```python
from build123d import *

# Parameters (mm, degrees)
BOSS_EXTRUDE1_DEPTH      = 12
BOSS_EXTRUDE1_DEPTH_BACK = 2
CUT_EXTRUDE1_DEPTH       = 5
SKETCH5_R                = 1
CUT_EXTRUDE2_DEPTH       = 7.26
CUT_EXTRUDE2_DEPTH_BACK  = 8.74
SKETCH6_R                = 1.95
CUT_EXTRUDE3_DEPTH       = 1.55
CUT_EXTRUDE4_DEPTH       = 2.5


with BuildPart() as part:
    # Sketch1 → Boss-Extrude1 (new body, two sides)
    with BuildSketch(Plane(origin=(0, 0, 0), x_dir=(1, 0, 0), z_dir=(0, 1, 0))) as boss_extrude1_sk:
        with BuildLine():
            Line((4.642363604, -4.565370009), (-4.68242218, -4.565370009))
            Line((-4.68242218, -4.565370009), (-2.520029288, -11.638238463))
            Line((-2.520029288, -11.638238463), (-2.520029288, -16.559323376))
            ThreePointArc((-2.520029288, -16.559323376), (-1.744780523, -16.658855879), (-0.965732534, -16.722114069))
            Line((-0.965732534, -16.722114069), (-0.020029288, -19.815370009))
            Line((-0.020029288, -19.815370009), (0.924969464, -16.724418368))
            ThreePointArc((0.924969464, -16.724418368), (1.704326405, -16.663043233), (2.479970712, -16.565370009))
            Line((2.479970712, -16.565370009), (2.479970712, -11.638238463))
            Line((2.479970712, -11.638238463), (4.642363604, -4.565370009))
        make_face()
    extrude(amount=BOSS_EXTRUDE1_DEPTH)
    extrude(boss_extrude1_sk.sketch, amount=-BOSS_EXTRUDE1_DEPTH_BACK)

    # Sketch2 → Cut-Extrude1 (cut)
    with BuildSketch(Plane(origin=(0, 0, 4.565370009), x_dir=(-1, 0, 0), z_dir=(0, 0, -1))):
        with BuildLine():
            Line((-2.878246061, 5.95), (2.918304637, 5.95))
            ThreePointArc((2.918304637, 5.95), (0.020029288, 8.05), (-2.878246061, 5.95))
        make_face()
        with BuildLine():
            Line((-2.878246061, 4.05), (2.918304637, 4.05))
            ThreePointArc((2.918304637, 4.05), (0.020029288, 1.95), (-2.878246061, 4.05))
        make_face()
    extrude(amount=-CUT_EXTRUDE1_DEPTH, mode=Mode.SUBTRACT)

    # Sketch5 → Cut-Extrude2 (cut, two sides)
    with BuildSketch(Plane(origin=(0, 5.74, 0), x_dir=(1, 0, 0), z_dir=(0, 1, 0))) as cut_extrude2_sk:
        with Locations((0, -7.065370009)):
            Circle(SKETCH5_R)
    extrude(amount=CUT_EXTRUDE2_DEPTH, mode=Mode.SUBTRACT)
    extrude(cut_extrude2_sk.sketch, amount=-CUT_EXTRUDE2_DEPTH_BACK, mode=Mode.SUBTRACT)

    # Sketch6 → Cut-Extrude3 (cut)
    with BuildSketch(Plane(origin=(0, 12, 0), x_dir=(1, 0, 0), z_dir=(0, 1, 0))):
        with Locations((0, -7.065370009)):
            Circle(SKETCH6_R)
    extrude(amount=-CUT_EXTRUDE3_DEPTH, mode=Mode.SUBTRACT)

    # Sketch7 → Cut-Extrude4 (cut)
    with BuildSketch(Plane(origin=(0, 12, 0), x_dir=(1, 0, 0), z_dir=(0, 1, 0))):
        Polygon((0.924969464, -16.724418368), (-0.020029288, -19.815370009), (-0.965732534, -16.722114069), align=None)
    cut_extrude4 = extrude(amount=-CUT_EXTRUDE4_DEPTH, mode=Mode.SUBTRACT)

    # Mirror1: Cut-Extrude4 across plane
    add(cut_extrude4.mirror(Plane.ZX.offset(5)), mode=Mode.SUBTRACT)


solid = part.part
```
Could you check a few things on this model? Use its own coordinates, in mm. A direction names the side the tool comes from. Round coordinates to 2 decimals unless told otherwise and drop trailing zeros. Loops run counter-clockwise (first coordinate to the right, second up) from the corner with the lowest first, then second, coordinate; pieces in that order, holes last. Notation, with made-up numbers: (59.5, -12.5) - (93.5, -12.5) arc R29 cw to (93.5, 9.5) - close; hole circle Ø4 at (-10.5, 88.5). An arc over 180 degrees is marked (long way). Answer as CSV lines item,"result".
1. I want a section at C-C on x = -1.25. List the corners of the cut face in (y, z) for me.
Filled in:
outline,"(-2, 4.57) - (2.21, 4.57) - (2.21, 9.57) - (4.05, 9.57) - (4.05, 4.57) - (5.95, 4.57) - (5.95, 9.57) - (7.79, 9.57) - (7.79, 4.57) - (12, 4.57) - (12, 5.57) - (10.45, 5.57) - (10.45, 8.56) - (12, 8.56) - (12, 16.7) - (-2, 16.7) - close"
2. I want a section at A-A on z = 9.25. List the corners of the cut face in (x, y) for me, then the cut area to 3 significant figures.
Filled in:
outline,"(-3.25, -2) - (3.21, -2) - (3.21, 12) - (-3.25, 12) - close; hole (-2.92, 4.05) arc R3.05 ccw to (2.88, 4.05) - close; hole (-2.92, 5.95) - (2.88, 5.95) arc R3.05 ccw to start"
area,"72.6 mm^2"
3. On a 3-axis mill with a long thin cutter (end or side, diameter ignored), from which of +Z, -Z, +X, -X, +Y, -Y can I reach the whole of each face in a straight line? I mean faces 1 (the face through (-0.42, 11.24, 8.97)), 2 (the face through (0, 3, 9.565)), 3 (the face through (2.48, 5, 14)). Say none if no direction works.
Filled in:
face 1,"+Y"
face 2,"-Z"
face 3,"+Z, +X, +Y, -Y"
4. I want a section at D-D on y = 6.5. List the corners of the cut face in (x, z) for me.
Filled in:
outline,"(-4.68, 4.57) - (-2.68, 4.57) - (-2.68, 9.57) - (2.64, 9.57) - (2.64, 4.57) - (4.64, 4.57) - (2.48, 11.64) - (2.48, 16.57) arc R16.75 ccw to (0.92, 16.72) - (-0.02, 19.82) - (-0.97, 16.72) arc R16.75 ccw to (-2.52, 16.56) - (-2.52, 11.64) - close"
5. I want a section at B-B on y = 10.25. List the corners of the cut face in (x, z) for me, then the cut area to 3 significant figures.
Filled in:
outline,"(-4.68, 4.57) - (4.64, 4.57) - (2.48, 11.64) - (2.48, 16.57) arc R16.75 ccw to (0.92, 16.72) - (-0.97, 16.72) arc R16.75 ccw to (-2.52, 16.56) - (-2.52, 11.64) - close; hole circle Ø2 at (0, 7.07)"
area,"72.7 mm^2"
6. Please list where these lines run through material, in increasing order: line 1 along Z through (x, y) = (0, 9.95); line 2 along Y through (x, z) = (-0.5, 8); line 3 along Y through (x, z) = (-2.25, 7.5). Write a range as [from, to].
Filled in:
line 1,"z = [4.57, 6.07], [8.07, 16.72]"
line 2,"y = [-2, 1.99], [4.05, 5.95], [8.01, 10.45]"
line 3,"y = [-2, 2.92], [4.05, 5.95], [7.08, 12]"
7. For pin 1 Ø1.6 at (x, z) = (0, 7.07) entering from +Y; pin 2 Ø2.5 at (y, z) = (7, 15) entering from +X; pin 3 Ø1.5 at (x, y) = (1, 10.5) entering from +Z; pin 4 Ø0.6 at (x, z) = (0, 18.5) entering from +Y, each with a flat end and sliding along its axis, tell me the tip position at first contact or that it passes through.
Filled in:
pin 1,"passes through"
pin 2,"stops at x = 2.48"
pin 3,"stops at z = 16.72"
pin 4,"stops at y = 9.5"
8. We'd pull the mould along Z, two halves only. Please class faces 4 (the face through (-0.5, 5.06, 18.25)), 5 (the face through (1, 10.45, 8)), 6 (the face through (0.461, 5.013, 7.953)), 7 (the face through (0, 4.05, 5.9)): +Z half, -Z half, draft (parallel to the pull), parting line (faces both ways), or undercut.
Filled in:
face 4,"+Z half"
face 5,"undercut"
face 6,"undercut"
face 7,"draft"
